Work out the finished part from the listing and answer in its coordinate system (mm). Face numbers are marked on the shaded views. Round coordinates to 2 decimals unless told otherwise and drop trailing zeros. Loops run counter-clockwise (first coordinate to the right, second up) from the corner with the lowest first, then second, coordinate; pieces in that order, holes last. Notation, with made-up numbers: M 36.5,-13 L 54.5,-13 A22 ccw 54.5,21 Z; hole C -38,33 d8. An arc over 180 degrees is marked long. One line per item, written item: value.
```python
from build123d import *

# Parameters (mm, degrees)
ESQUISSE1_W        = 3.4
ESQUISSE1_H        = 6
BOSS_EXTRU_1_DEPTH = 1.9
ESQUISSE2_W        = 2.9
ESQUISSE2_H        = 0.2
R_VOLUTION1_ANGLE  = 40
ESQUISSE4_W        = 1
ESQUISSE4_H        = 2.9
BOSS_EXTRU_2_DEPTH = 0.19
CONG_1_R           = 0.1
CONG_2_R           = 0.05
ESQUISSE6_W        = 0.7
ESQUISSE6_H        = 0.2
R_VOLUTION2_ANGLE  = 46
ESQUISSE8_W        = 1
ESQUISSE8_H        = 0.7
BOSS_EXTRU_3_DEPTH = 0.2
CONG_3_R           = 0.1
CONG_4_R           = 0.05


with BuildPart() as part:
    # Esquisse1 → Boss.-Extru.1 (new body)
    with BuildSketch(Plane(origin=(0, 0, 0), x_dir=(1, 0, 0), z_dir=(0, 1, 0))):
        with Locations((1.7, 3)):
            Rectangle(ESQUISSE1_W, ESQUISSE1_H)
    extrude(amount=BOSS_EXTRU_1_DEPTH)

    # Esquisse2 → Révolution1 (revolve)
    with BuildSketch(Plane(origin=(3.4, 0, 0), x_dir=(0, 0, -1), z_dir=(1, 0, 0))):
        with Locations((3, 0.599818591)):
            Rectangle(ESQUISSE2_W, ESQUISSE2_H)
    revolve(axis=Axis((3.4, -1.500181409, -1.55), (0, 0, -1)), revolution_arc=R_VOLUTION1_ANGLE)

    # Esquisse4 → Boss.-Extru.2 (add)
    with BuildSketch(Plane(origin=(0, 0, 0), x_dir=(1, 0, 0), z_dir=(0, 1, 0))):
        with Locations((5.185575219, 3)):
            Rectangle(ESQUISSE4_W, ESQUISSE4_H)
    extrude(amount=BOSS_EXTRU_2_DEPTH)

    # Congé1
    # the kernel refuses this fillet: 0.1 mm, written as the material it adds along each edge
    with BuildSketch(Plane(origin=(4.685575219, 0.031907477, -4.45), x_dir=(-0.7735020248903554, 0.6337938288517173, 0), z_dir=(0, 0, 1))) as cong_1_piece_1:
        with BuildLine():
            CenterArc((0.04556478, 0.099993175), CONG_1_R, 228.861958966, 41.807458726)
            Line((-0.020222762, 0.024680498), (-0.021538513, 0.023174245))
            ThreePointArc((-0.021538513, 0.023174245), (-0.011658385, 0.011072661), (-0.001547004, -0.001267588))
            Line((-0.001547004, -0.001267588), (-2.3367e-05, -0.001999863))
            ThreePointArc((-2.3367e-05, -0.001999863), (0.023366554, -0.002136504), (0.046756475, -0.001999863))
            Line((0.046756475, -0.001999863), (0.046733108, 0))
        make_face()
    extrude(amount=2.9)
    with BuildSketch(Plane(origin=(4.808292159, 0.19, -1.55), x_dir=(-0.7733264230058849, 0.6340080784035191, 0), z_dir=(0, 0, -1))) as cong_1_piece_2:
        with BuildLine():
            CenterArc((0.035756325, 0.099996843), CONG_1_R, 230.653545738, 38.8911858)
            Line((-0.027644483, 0.022664201), (-0.028912499, 0.021117548))
            Line((-0.028912499, 0.021117548), (-0.001268016, -0.001546653))
            Line((-0.001268016, -0.001546653), (1.5892e-05, -0.001999937))
            ThreePointArc((1.5892e-05, -0.001999937), (0.01748087, -0.001930549), (0.034945848, -0.001999937))
            Line((0.034945848, -0.001999937), (0.03496174, 0))
        make_face()
    extrude(amount=2.9)

    # Congé2
    cong_2_edges = [part.edges().sort_by_distance(p)[0] for p in [
        (5.264807437, 0.19, -4.45),
        (5.685575219, 0.19, -3),
        (5.264807437, 0.19, -1.55),
        (4.132405504, 0.574326286, -4.45),
        (4.132405504, 0.574326286, -1.55),
        (4.810748495, 0.195704196, -1.55),
        (4.810748495, 0.195704196, -4.45),
    ]]
    fillet(cong_2_edges, radius=CONG_2_R)

    # Esquisse6 → Révolution2 (revolve)
    with BuildSketch(Plane.ZY):
        with Locations((-3, 0.599818591)):
            Rectangle(ESQUISSE6_W, ESQUISSE6_H)
        with Locations((-5.2, 0.599818591)):
            Rectangle(ESQUISSE6_W, ESQUISSE6_H)
        with Locations((-0.8, 0.599818591)):
            Rectangle(ESQUISSE6_W, ESQUISSE6_H)
    revolve(axis=Axis((0, -1, -6), (0, 0, 1)), revolution_arc=R_VOLUTION2_ANGLE)

    # Esquisse8 → Boss.-Extru.3 (add)
    with BuildSketch(Plane(origin=(0, 0, 0), x_dir=(1, 0, 0), z_dir=(0, 1, 0))):
        with Locations((-1.578879206, 0.8)):
            Rectangle(ESQUISSE8_W, ESQUISSE8_H)
        with Locations((-1.578879206, 3)):
            Rectangle(ESQUISSE8_W, ESQUISSE8_H)
        with Locations((-1.578879206, 5.2)):
            Rectangle(ESQUISSE8_W, ESQUISSE8_H)
    extrude(amount=BOSS_EXTRU_3_DEPTH)

    # Congé3
    cong_3_edges = [part.edges().sort_by_distance(p)[0] for p in [
        (-1.078879206, 0.041861538, -0.8),
        (-1.203903336, 0.2, -0.8),
        (-1.203903336, 0.2, -3),
        (-1.203903336, 0.2, -5.2),
        (-1.078879206, 0.041861538, -3),
        (-1.078879206, 0.041861538, -5.2),
    ]]
    fillet(cong_3_edges, radius=CONG_3_R)

    # Congé4
    cong_4_edges = [part.edges().sort_by_distance(p)[0] for p in [
        (-2.078879206, 0.2, -0.8),
        (-1.661803435, 0.2, -0.45),
        (-2.078879206, 0.2, -3),
        (-1.661803435, 0.2, -2.65),
        (-2.078879206, 0.2, -5.2),
        (-1.661803435, 0.2, -4.85),
        (-0.633401975, 0.577398231, -1.15),
        (-0.633401975, 0.577398231, -0.45),
        (-1.661803435, 0.2, -1.15),
        (-0.633401975, 0.577398231, -5.55),
        (-0.633401975, 0.577398231, -4.85),
        (-1.661803435, 0.2, -5.55),
        (-0.633401975, 0.577398231, -3.35),
        (-0.633401975, 0.577398231, -2.65),
        (-1.661803435, 0.2, -3.35),
        (-1.207464749, 0.207201966, -0.45),
        (-1.207464749, 0.207201966, -1.15),
        (-1.207464749, 0.207201966, -4.85),
        (-1.207464749, 0.207201966, -5.55),
        (-1.207464749, 0.207201966, -2.65),
        (-1.207464749, 0.207201966, -3.35),
    ]]
    fillet(cong_4_edges, radius=CONG_4_R)


solid = part.part
```
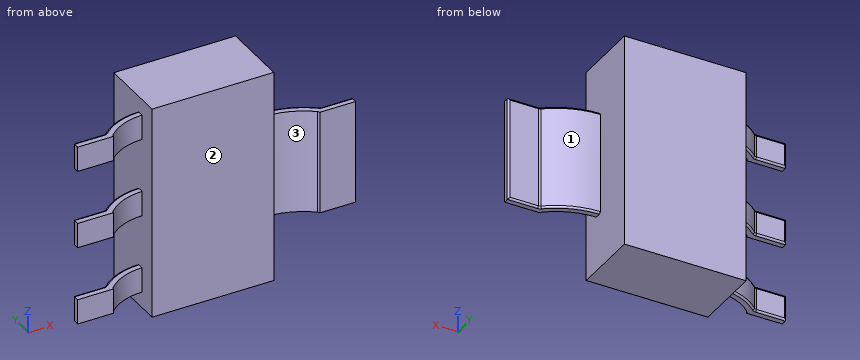
1) Find section D-D (y = 1.2). Give the vertices of the cut face in (x, z), then the cut area to 3 significant figures.
Check values:
outline: M 0,-6 L 3.4,-6 L 3.4,0 L 0,0 Z
area: 20.4 mm2
2) Find the intervals of material crossed by probe 1 along X at (y, z) = (1.5, -0.4); probe 2 along Y at (x, z) = (5.25, -1.8); probe 3 along Y at (x, z) = (-0.75, -3.1), in increasing order. Write a range as from..to.
Check values:
probe 1: 0..3.4
probe 2: 0..0.19
probe 3: 0.3..0.53
3) Each of these flat-tipped pins is pushed along its axis until it touches: pin 1 (0.5 mm diameter, centred on x = -1, y = 0.5, fed in from +Z); pin 2 (0.9 mm diameter, centred on x = 5, z = -3, fed in from +Y); pin 3 (0.5 mm diameter, centred on x = -1.5, z = -1, fed in from +Y). Where does it stop, or does it pass through?
Check values:
pin 1: z = -0.45
pin 2: y = 0.38
pin 3: y = 0.2
4) Find section B-B (x = -0.25). Give the number of separate pieces and of enclosed holes in the cut face, then the cut area to 3 significant figures.
Check values:
separate pieces: 3
enclosed holes: 0
area: 0.422 mm2
5) The mould has two halves that part along X. Classify the marked faces 1, 2 and 3: +X half, -X half, draft (parallel to the pull), parting line (faces both ways), or undercut.
Check values:
face 1: +X half
face 2: draft
face 3: undercut
6) Find section A-A (z = -2.25). Give the vertices of the cut face in (x, y), then the cut area to 3 significant figures.
Check values:
outline: M 0,0 L 3.4,0 L 3.4,0.5 A2 cw 4.65,0.06 A0.1 cw 4.69,0 L 5.69,0 L 5.69,0.14 A0.05 ccw 5.64,0.19 L 4.84,0.19 A0.1 cw 4.78,0.21 A2.2 ccw 3.4,0.7 L 3.4,1.9 L 0,1.9 Z
area: 6.93 mm2
